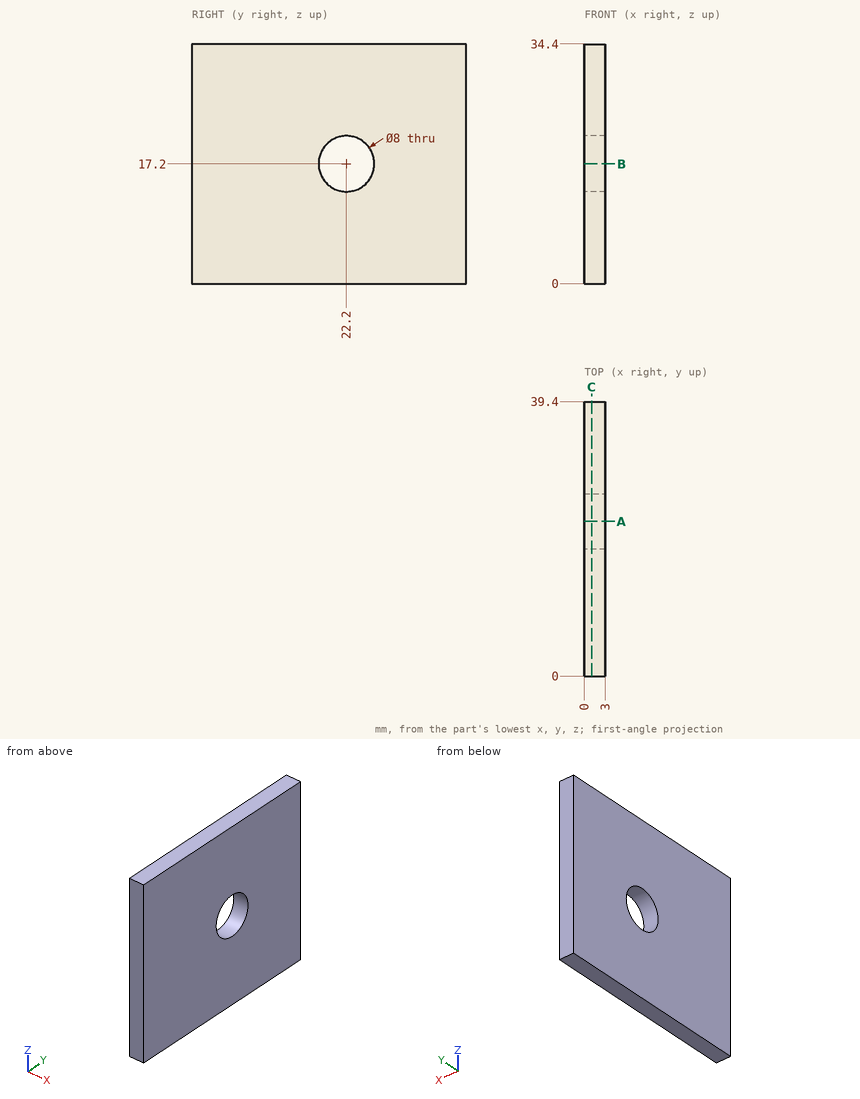
Source: three-view drawing plus pictorial views. Frame: mm from the lowest corner of the part. Give positions to 0.01 mm unless a question says otherwise; leave off trailing zeros. Order: outer loops, then holes, each group sorted by start corner. A loop starts at its lowest first (then second) coordinate and runs counter-clockwise, first axis right, second up. Notation, with made-up numbers: M -33.5,83.25 L 13.5,83.25 A25 ccw 13.5,117.25 Z; hole C -12,73 d5. An arc over 180 degrees is marked long. One line per question, with ' | ' between items. Start each with the question number.
1. Section query C-C (x = 1.05). Return the cut outline in (y, z), and give its area (3 significant figures).
2. First-contact query: pin 1 Ø10 at (y, z) = (17.5, 23) entering from -X. Flat tip, straight axial feed; report the tip coordinate or a pass-through.
3. Section query B-B (z = 17.2). Return the cut outline in (x, y).
4. Section query A-A (y = 22.2). Return the cut outline in (x, z), and give its area (3 significant figures).
5. Material intervals for probe 1 along Z at (x, y) = (1.65, 22.2); probe 2 along Z at (x, y) = (0.3, 21), sorted ascending. Write a range as [from, to].
Here are the results:
1) outline: M 0,0 L 39.4,0 L 39.4,34.4 L 0,34.4 Z; hole C 22.2,17.2 d8 | area: 1,310 mm²
2) pin 1: x = 0
3) outline: M 0,0 L 3,0 L 3,18.2 L 0,18.2 Z; M 0,26.2 L 3,26.2 L 3,39.4 L 0,39.4 Z
4) outline: M 0,0 L 3,0 L 3,13.2 L 0,13.2 Z; M 0,21.2 L 3,21.2 L 3,34.4 L 0,34.4 Z | area: 79.2 mm²
5) probe 1: [0, 13.2], [21.2, 34.4] | probe 2: [0, 13.38], [21.02, 34.4]
